Answer from the drawing. Dimensions are ordinates in mm from the lowest x, y and z of the part. A direction names the side the tool comes from. Round coordinates to 2 decimals unless told otherwise and drop trailing zeros. Order: outer loops, then holes, each group sorted by start corner. A loop starts at its lowest first (then second) coordinate and runs counter-clockwise, first axis right, second up. Notation, with made-up numbers: M -13,1.5 L 7,1.5 A17 ccw 7,16.5 Z; hole C 49,19.5 d4. An arc over 180 degrees is marked long. Use one line per item in the form item = value. Start each with the question number.
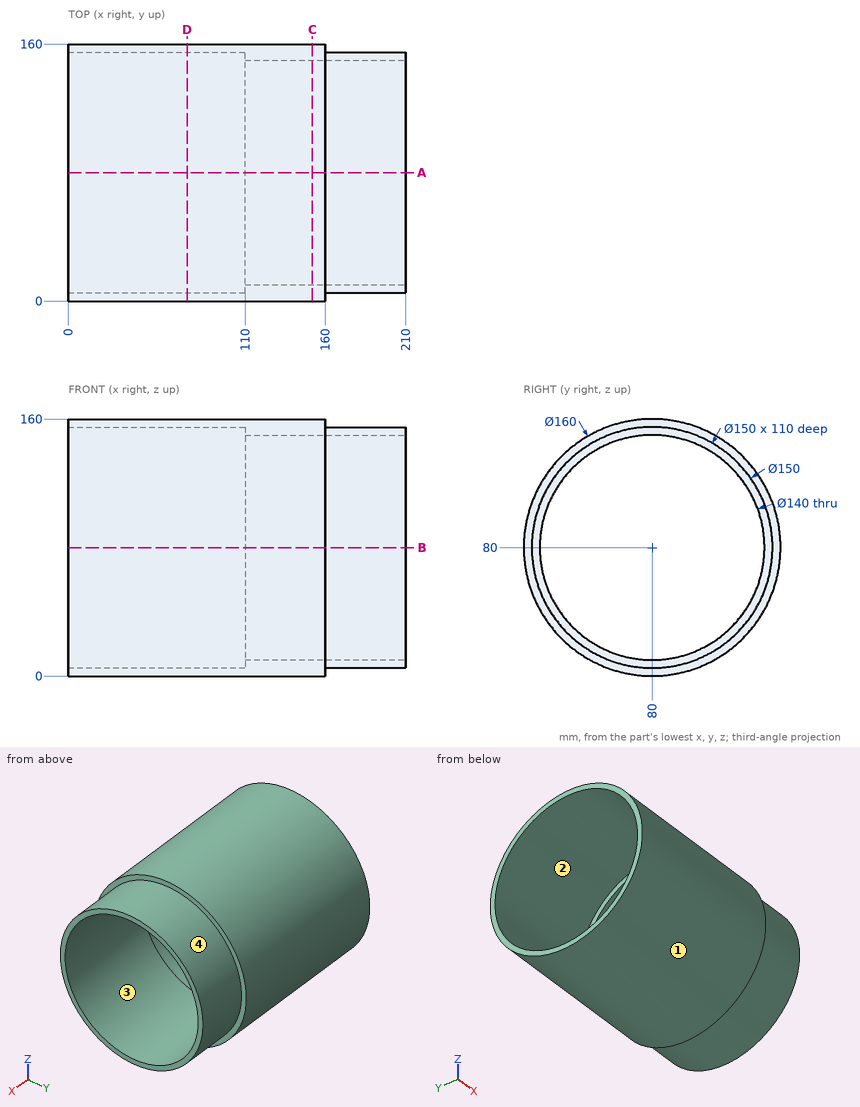
Item 1: Section D-D (x = 74) is taken. Write down the section's boundary in (y, z).
Item 2: Section A-A (y = 80) is taken. Write down the section's boundary in (x, z).
Item 3: Given P1, Ø3, axis at x = 60.5, z = 20, coming from the -Y side; P2, Ø2, axis at x = 183, z = 83, coming from the -Y side; P3, Ø1.5, axis at x = 102, y = 76.5, coming from the +Z side, each flat-ended and moving along its own axis, determine where each tip first touches the part or whether it passes through.
Item 4: Find the intervals of material crossed by L1, parallel to Y at x = 41, z = 78.5 (3 decimals); L2, parallel to Y at x = 138, z = 79; L3, parallel to X at y = 144, z = 33, in increasing order. Write a range as [from, to].
Item 5: Section C-C (x = 152) is taken. Write down the section's boundary in (y, z), and give its area (3 significant figures).
Item 6: A tool of negligible diameter and unlimited length cuts with its end or side. For the marked faces 3 and 4, from which of +Z, -Z, +X, -X, +Y, -Y can it reach the whole face along a straight path? Write none if from no direction.
Item 7: For a pull along Y with two mould halves and no side action, classify the marked faces 1 and 2 as pulls with the +Y half, pulls with the -Y half, needs draft (parallel to the pull), parting line crosses it, or undercut.
The answers:
q1.outline = C 80,80 d160; hole C 80,80 d150
q2.outline = M 0,0 L 160,0 L 160,5 L 210,5 L 210,10 L 110,10 L 110,5 L 0,5 Z; M 0,155 L 110,155 L 110,150 L 210,150 L 210,155 L 160,155 L 160,160 L 0,160 Z
q3.P1 = 25.43
q3.P2 = 5.03
q3.P3 = 159.95
q4.L1 = [0.014, 5.015], [154.985, 159.986]
q4.L2 = [0.01, 10.01], [149.99, 159.99]
q4.L3 = [0, 160]
q5.outline = C 80,80 d160; hole C 80,80 d140
q5.area = 4,710 mm²
q6.face_3 = +X, -X
q6.face_4 = +X
q7.face_1 = parting line crosses it
q7.face_2 = undercut
